Verification items for the finished model (mm, model axes). Give positions to 0.01 mm unless a question says otherwise; leave off trailing zeros. Order: outer loops, then holes, each group sorted by start corner. A loop starts at its lowest first (then second) coordinate and runs counter-clockwise, first axis right, second up.
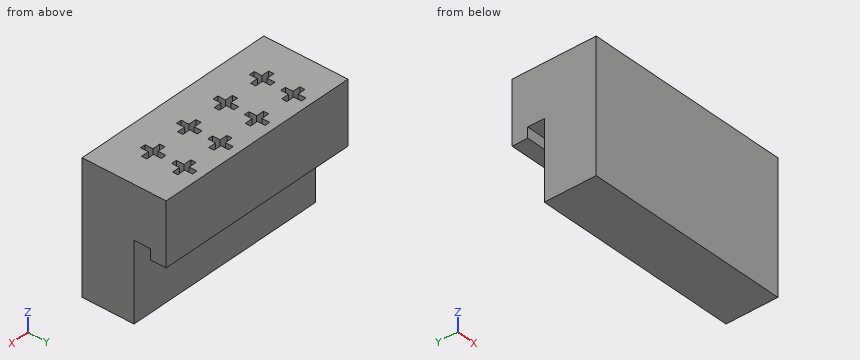
from build123d import *

# Parameters (mm, degrees)
BOSS_EXTRUDE1_DEPTH = 40
CUT_EXTRUDE3_DEPTH  = 8


with BuildPart() as part:
    # Sketch1 → Boss-Extrude1 (new body)
    with BuildSketch(Plane(origin=(0, 0, 0), x_dir=(0, 0, -1), z_dir=(1, 0, 0))):
        Polygon((-9.638596491, 6.2), (2.361403509, 6.2), (2.361403509, 3.2), (0.361403509, 3.2), (0.361403509, 0), (15.361403509, 0), (15.361403509, -10), (-9.638596491, -10), align=None)
    extrude(amount=BOSS_EXTRUDE1_DEPTH)

    # Sketch2 → Cut-Extrude3 (cut)
    with BuildSketch(Plane.XY.offset(9.638596491)):
        Polygon((14, 2.2), (14, 3.2), (15.5, 3.2), (15.5, 4.7), (16.5, 4.7), (16.5, 3.2), (18, 3.2), (18, 2.2), (16.5, 2.2), (16.5, 0.7), (15.5, 0.7), (15.5, 2.2), align=None)
        Polygon((14.051371054, -3.758215043), (14.051371054, -2.758215043), (15.551371054, -2.758215043), (15.551371054, -1.258215043), (16.551371054, -1.258215043), (16.551371054, -2.758215043), (18.051371054, -2.758215043), (18.051371054, -3.758215043), (16.551371054, -3.758215043), (16.551371054, -5.258215043), (15.551371054, -5.258215043), (15.551371054, -3.758215043), align=None)
        Polygon((22.051371054, -3.808568011), (22.051371054, -2.808568011), (23.551371054, -2.808568011), (23.551371054, -1.308568011), (24.551371054, -1.308568011), (24.551371054, -2.808568011), (26.051371054, -2.808568011), (26.051371054, -3.808568011), (24.551371054, -3.808568011), (24.551371054, -5.308568011), (23.551371054, -5.308568011), (23.551371054, -3.808568011), align=None)
        Polygon((22, 2.149647032), (22, 3.149647032), (23.5, 3.149647032), (23.5, 4.649647032), (24.5, 4.649647032), (24.5, 3.149647032), (26, 3.149647032), (26, 2.149647032), (24.5, 2.149647032), (24.5, 0.649647032), (23.5, 0.649647032), (23.5, 2.149647032), align=None)
        Polygon((30, 2.2), (30, 3.2), (31.5, 3.2), (31.5, 4.7), (32.5, 4.7), (32.5, 3.2), (34, 3.2), (34, 2.2), (32.5, 2.2), (32.5, 0.7), (31.5, 0.7), (31.5, 2.2), align=None)
        Polygon((30.051371054, -3.758215043), (30.051371054, -2.758215043), (31.551371054, -2.758215043), (31.551371054, -1.258215043), (32.551371054, -1.258215043), (32.551371054, -2.758215043), (34.051371054, -2.758215043), (34.051371054, -3.758215043), (32.551371054, -3.758215043), (32.551371054, -5.258215043), (31.551371054, -5.258215043), (31.551371054, -3.758215043), align=None)
        Polygon((6, 2.2), (6, 3.2), (7.5, 3.2), (7.5, 4.7), (8.5, 4.7), (8.5, 3.2), (10, 3.2), (10, 2.2), (8.5, 2.2), (8.5, 0.7), (7.5, 0.7), (7.5, 2.2), align=None)
        Polygon((6.051371054, -2.758215043), (7.551371054, -2.758215043), (7.551371054, -1.258215043), (8.551371054, -1.258215043), (8.551371054, -2.758215043), (10.051371054, -2.758215043), (10.051371054, -3.758215043), (8.551371054, -3.758215043), (8.551371054, -5.258215043), (7.551371054, -5.258215043), (7.551371054, -3.758215043), (6.051371054, -3.758215043), align=None)
    extrude(amount=-CUT_EXTRUDE3_DEPTH, mode=Mode.SUBTRACT)


solid = part.part
(1) Section check C-C, the plane z = 6. Give the number of separate pieces and of enclosed holes in the cut face, then the cut area to 3 significant figures.
Solved:
separate pieces: 1
enclosed holes: 8
area: 592 mm2
(2) Section check B-B, the plane y = 3.75. Enter the section's corners in (x, z), then the cut area to 3 significant figures.
Solved:
outline: (0, -2.36) - (40, -2.36) - (40, 9.64) - (32.5, 9.64) - (32.5, 1.64) - (31.5, 1.64) - (31.5, 9.64) - (24.5, 9.64) - (24.5, 1.64) - (23.5, 1.64) - (23.5, 9.64) - (16.5, 9.64) - (16.5, 1.64) - (15.5, 1.64) - (15.5, 9.64) - (8.5, 9.64) - (8.5, 1.64) - (7.5, 1.64) - (7.5, 9.64) - (0, 9.64) - close
area: 448 mm2
(3) Go/stop test with a flat-tipped pin: pin 1 (2 mm diameter, centred on x = 17, z = -6, fed in from +Y). Record where the tip stops, or that it passes through.
Solved:
pin 1: stops at y = 0
(4) Section check D-D, the plane x = 17.5. Enter the section's corners in (y, z).
Solved:
outline: (-10, -15.36) - (0, -15.36) - (0, -0.36) - (3.2, -0.36) - (3.2, -2.36) - (6.2, -2.36) - (6.2, 9.64) - (3.2, 9.64) - (3.2, 1.64) - (2.2, 1.64) - (2.2, 9.64) - (-2.76, 9.64) - (-2.76, 1.64) - (-3.76, 1.64) - (-3.76, 9.64) - (-10, 9.64) - close
(5) Scan lines: line 1 (Y direction, x = 16, z = 7.75); line 2 (X direction, y = 2.25, z = 3.5); line 3 (X direction, y = 0.75, z = 2.25). Record each from-to range of solid material in increasing order.
Solved:
line 1: y = -10 to -5.26, -1.26 to 0.7, 4.7 to 6.2
line 2: x = 0 to 6, 10 to 14, 18 to 22, 26 to 30, 34 to 40
line 3: x = 0 to 7.5, 8.5 to 15.5, 16.5 to 23.5, 24.5 to 31.5, 32.5 to 40
(6) Section check A-A, the plane x = 37. Enter the section's corners in (y, z), then the cut area to 3 significant figures.
Solved:
outline: (-10, -15.36) - (0, -15.36) - (0, -0.36) - (3.2, -0.36) - (3.2, -2.36) - (6.2, -2.36) - (6.2, 9.64) - (-10, 9.64) - close
area: 318 mm2
